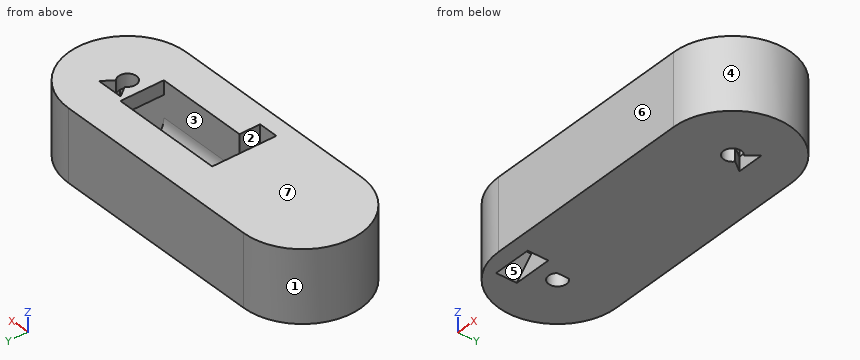
from build123d import *

# Parameters (mm, degrees)
SALIENTE_EXTRUIR1_DEPTH = 40
CORTAR_EXTRUIR2_DEPTH   = 10
CORTAR_EXTRUIR4_DEPTH   = 20
CROQUIS6_R              = 12.2
CORTAR_EXTRUIR6_DEPTH   = 63
CROQUIS7_W              = 24.4
CROQUIS7_H              = 24.4
CORTAR_EXTRUIR9_DEPTH   = 30
CROQUIS8_W              = 12.2
CROQUIS8_H              = 11.6
CORTAR_EXTRUIR10_DEPTH  = 50
CORTAR_EXTRUIR11_REACH  = 123.586
CROQUIS9_W              = 11.6
CROQUIS9_H              = 11.6
CHAFL_N1_SIZE           = 10


with BuildPart() as part:
    # Croquis1 → Saliente-Extruir1 (new body)
    with BuildSketch(Plane.XY):
        with BuildLine():
            Line((76.972889038, 33), (-43.027110962, 33))
            ThreePointArc((-43.027110962, 33), (-76.027110962, 0), (-43.027110962, -33))
            Line((-43.027110962, -33), (76.972889038, -33))
            ThreePointArc((76.972889038, -33), (109.972889038, 0), (76.972889038, 33))
        make_face()
        with BuildLine():
            Line((69.472889038, 10), (84.472889038, 10))
            Line((84.472889038, 10), (79.972889038, 4))
            ThreePointArc((79.972889038, 4), (76.972889038, -5), (73.972889038, 4))
            Line((73.972889038, 4), (69.472889038, 10))
        make_face(mode=Mode.SUBTRACT)
    extrude(amount=SALIENTE_EXTRUIR1_DEPTH)

    # Croquis1<4> → Cortar-Extruir2 (cut)
    with BuildSketch(Plane.XY):
        with BuildLine():
            Line((-39.234058455, -3.257722008), (-39.234058455, 3.257722008))
            ThreePointArc((-39.234058455, 3.257722008), (-48.027110962, 0), (-39.234058455, -3.257722008))
        make_face()
    extrude(amount=CORTAR_EXTRUIR2_DEPTH, mode=Mode.SUBTRACT)

    # Croquis5 → Cortar-Extruir4 (cut)
    with BuildSketch(Plane.XY.offset(40)):
        Polygon((66.972889038, -12.2), (66.972889038, 12.2), (3.972889038, 12.2), (3.972889038, -23.8), (15.110447518, -23.8), (15.110447518, -12.2), align=None)
    extrude(amount=-CORTAR_EXTRUIR4_DEPTH, mode=Mode.SUBTRACT)

    # Croquis6 → Cortar-Extruir6 (cut)
    with BuildSketch(Plane(origin=(3.972889038, 0, 0), x_dir=(0, 0, -1), z_dir=(1, 0, 0))):
        with Locations((-20, 0)):
            Circle(CROQUIS6_R)
        with BuildLine():
            ThreePointArc((-20, -12.2), (-32.2, 0), (-20, 12.2))
            Line((-20, 12.2), (-40, 12.2))
            Line((-40, 12.2), (-40, -12.2))
            Line((-40, -12.2), (-20, -12.2))
        make_face()
    extrude(amount=CORTAR_EXTRUIR6_DEPTH, mode=Mode.SUBTRACT)

    # Croquis7 → Cortar-Extruir9 (cut)
    with BuildSketch(Plane.ZY.offset(-66.972889038)):
        with Locations((20, 0)):
            Rectangle(CROQUIS7_W, CROQUIS7_H)
    extrude(amount=-CORTAR_EXTRUIR9_DEPTH, mode=Mode.SUBTRACT)

    # Croquis8 → Cortar-Extruir10 (cut)
    with BuildSketch(Plane(origin=(3.972889038, 0, 0), x_dir=(0, 0, -1), z_dir=(1, 0, 0))):
        with Locations((-26.1, -18)):
            Rectangle(CROQUIS8_W, CROQUIS8_H)
    extrude(amount=-CORTAR_EXTRUIR10_DEPTH, mode=Mode.SUBTRACT)

    # Croquis9 → Cortar-Extruir11 (cut, up to next)
    with BuildSketch(Plane(origin=(0, 0, 0), x_dir=(-1, 0, 0), z_dir=(0, 0, -1)), mode=Mode.PRIVATE) as cortar_extruir11_sk1:
        with Locations((40.227110962, -18)):
            Rectangle(CROQUIS9_W, CROQUIS9_H)
    cortar_extruir11_tool1 = extrude(cortar_extruir11_sk1.sketch, amount=-CORTAR_EXTRUIR11_REACH, mode=Mode.PRIVATE) & part.part
    add(cortar_extruir11_tool1.solids().sort_by_distance((-40.227111, -18, 0))[0], mode=Mode.SUBTRACT)

    # Chaflán1
    chafl_n1_edges = [part.edges().sort_by_distance(p)[0] for p in [
        (-46.027110962, -18, 0),
    ]]
    chamfer(chafl_n1_edges, length=CHAFL_N1_SIZE)


solid = part.part
Read the model definition and answer for the solid it produces. Units are mm, in the model's axes. Face numbers are marked on the shaded views. A direction names the side the tool comes from. Coordinates: 2 decimals unless noted, no trailing zeros. Loops run counter-clockwise (first coordinate to the right, second up) from the corner with the lowest first, then second, coordinate; pieces in that order, holes last. Notation, with made-up numbers: (27, -30.75) -> (85, -30.75) arc R19 ccw to (85, -12.75) -> close; hole circle Ø8 at (30, -20.5). An arc over 180 degrees is marked (long way). Write item = value, one per line. Start each with the question number.
1) The part is cut by section C-C, the plane x = 27.5. Determine the outline of the cut face in (y, z), plus the area to 3 significant figures.
2) The part is cut by section A-A, the plane x = -31.5. Determine the outline of the cut face in (y, z).
3) The mould has two halves that part along Y. Classify the marked faces 4, 5, 6 and 7: pulls with the +Y half, pulls with the -Y half, needs draft (parallel to the pull), parting line crosses it, or undercut.
4) For the marked faces 1, 2 and 3, determine the directions among +Z, -Z, +X, -X, +Y, -Y from which every point of the face is accessible in a straight line to the end or side of a thin tool.
5) The part is cut by section B-B, the plane z = 28.5. Determine the outline of the cut face in (x, y).
6) Find the intervals of material crossed by L1, parallel to X at y = 0, z = 2.5; L2, parallel to X at y = 0, z = 8; L3, parallel to Y at x = -43, z = 5, in increasing order. Write a range as from..to.
7) The part is cut by section D-D, the plane y = -8. Determine the outline of the cut face in (x, z), plus the area to 3 significant figures.
8) Given P1, Ø7.5, axis at y = 2.5, z = 26, coming from the -X side; P2, Ø8, axis at x = 91, y = -10, coming from the -Z side; P3, Ø6, axis at y = -19, z = 25.5, coming from the +X side; P4, Ø6, axis at y = -16, z = 8, coming from the -X side, each flat-ended and moving along its own axis, determine where each tip first touches the part or whether it passes through.
Result:
q1.outline = (-33, 0) -> (33, 0) -> (33, 40) -> (12.2, 40) -> (12.2, 20) arc R12.2 cw to (-12.2, 20) -> (-12.2, 40) -> (-33, 40) -> close
q1.area = 1,920 mm²
q2.outline = (-33, 0) -> (33, 0) -> (33, 40) -> (-33, 40) -> close; hole (-23.8, 20) -> (-12.2, 20) -> (-12.2, 32.2) -> (-23.8, 32.2) -> close
q3.face_4 = parting line crosses it
q3.face_5 = undercut
q3.face_6 = pulls with the -Y half
q3.face_7 = needs draft
q4.face_1 = +Z, -Z, -X
q4.face_2 = +Z
q4.face_3 = none
q5.outline = (-43.03, -33) -> (76.97, -33) arc R33 ccw to (76.97, 33) -> (-43.03, 33) arc R33 ccw to start; hole (-46.03, -23.8) -> (15.11, -23.8) -> (15.11, -12.2) -> (96.97, -12.2) -> (96.97, 12.2) -> (3.97, 12.2) -> (3.97, -12.2) -> (-46.03, -12.2) -> close
q6.L1 = -76.03..-48.03, -39.23..71.97, 81.97..109.97
q6.L2 = -76.03..-48.03, -39.23..3.97, 96.97..109.97
q6.L3 = -33..-23.8, -12.2..-5, 5..33
q7.outline = (-75.04, 0) -> (108.99, 0) -> (108.99, 40) -> (66.97, 40) -> (66.97, 32.2) -> (96.97, 32.2) -> (96.97, 7.8) -> (66.97, 7.8) -> (66.97, 10.79) -> (3.97, 10.79) -> (3.97, 40) -> (-75.04, 40) -> close
q7.area = 4,790 mm²
q8.P1 = -76.03
q8.P2 = 0
q8.P3 = 105.83
q8.P4 = -73.36
